Can you work these out from the model? Positions are in its coordinate system, mm. A direction names the side the tool comes from. Round coordinates to 2 decimals unless told otherwise and drop trailing zeros. Loops run counter-clockwise (first coordinate to the right, second up) from the corner with the lowest first, then second, coordinate; pieces in that order, holes last.
(1) I want a section at B-B on x = 76.2. Write out the boundary of the cut face in (y, z).
(2) Which directions (+Z, -Z, +X, -X, +Y, -Y) give clear straight access to the entire face, cutting with the end or side of a thin tool? Please do faces 1 (the face through (19, -58, 12.7)), 2 (the face through (0, -56, 6)), 3 (the face through (133, -58, 12.7)).
(3) Thinking about a two-plate mould opening in X: for faces 4 (the face through (114.3, -58, 52)), 5 (the face through (38.1, -58, 52)), 6 (the face through (75.495, -57.95, 59.858)), 7 (the face through (41, -56, 92.075)), which applies, released by +X, released by -X, zero draft, split by the parting line, or undercut?
(4) If I drill on line 1 along Z through (x, y) = (6, -105.5); line 2 along X through (y, z) = (-75, 27); line 3 along X through (y, z) = (-49, 71.5), over which ranges is the centre line in solid material (lowest first)?
(5) I want a section at C-C on z = 35. Write out the boundary of the cut face in (x, y), plus the area to 3 significant figures.
(6) Will these pins go through, and if not, where does the flat tip stop? pin 1 Ø1 at (y, z) = (-93, 21) entering from +X; pin 2 Ø11.5 at (x, y) = (134, -30) entering from +Z; pin 3 Ø1.5 at (x, y) = (98.5, -24) entering from +Z.
from build123d import *

# Parameters (mm, degrees)
F0_W     = 152.4
F0_H     = 92.075
F1_DEPTH = 114.3
F2_W     = 38.1
F2_H     = 79.375
F3_DEPTH = 114.301
F5_DEPTH = 114.301


with BuildPart() as f1:
    # F0 (on Front) → F1 (new body)
    with BuildSketch(Plane.XZ):
        with Locations((76.2, 46.0375)):
            Rectangle(F0_W, F0_H)
    extrude(amount=F1_DEPTH)

    # F2 (on face) → F3 (cut, through all)
    with BuildSketch(Plane.XZ.offset(114.3)):
        with Locations((19.05, 52.3875)):
            Rectangle(F2_W, F2_H)
        with Locations((133.35, 52.3875)):
            Rectangle(F2_W, F2_H)
    extrude(amount=-F3_DEPTH, mode=Mode.SUBTRACT)

    # F4 (on face) → F5 (cut, through all)
    with BuildSketch(Plane.XZ.offset(114.3)):
        with BuildLine():
            Line((107.95, 92.075), (44.45, 92.075))
            ThreePointArc((44.45, 92.075), (76.2, 59.849693), (107.95, 92.075))
        make_face()
    extrude(amount=-F5_DEPTH, mode=Mode.SUBTRACT)


solid = f1.part
Filled sheet:
1. outline: (-114.3, 0) - (0, 0) - (0, 59.85) - (-114.3, 59.85) - close
2. face 1: +Z, -X, +Y, -Y
2. face 2: +Z, -Z, -X, +Y, -Y
2. face 3: +Z, +X, +Y, -Y
3. face 4: released by +X
3. face 5: released by -X
3. face 6: undercut
3. face 7: zero draft
4. line 1: z = 0 to 12.7
4. line 2: x = 38.1 to 114.3
4. line 3: x = 38.1 to 51.62, 100.78 to 114.3
5. outline: (38.1, -114.3) - (114.3, -114.3) - (114.3, 0) - (38.1, 0) - close
5. area: 8,710 mm2
6. pin 1: stops at x = 114.3
6. pin 2: stops at z = 12.7
6. pin 3: stops at z = 69.76
